Check sheet for the modelled part. Datum: model origin and axes. Units: mm. Round coordinates to 2 decimals unless told otherwise and drop trailing zeros. Loops run counter-clockwise (first coordinate to the right, second up) from the corner with the lowest first, then second, coordinate; pieces in that order, holes last. Notation, with made-up numbers: (-1.75, -35.5) - (7.25, -35.5) arc R19 cw to (7.25, -2.5) - close; hole circle Ø7 at (58.5, 28). An arc over 180 degrees is marked (long way). Answer in a Markdown table with one row per item. Add a question column.
(1) Thickness scan on line 1 along Y through (x, z) = (4, 6.5); line 2 along Y through (x, z) = (-2, 2.5); line 3 along Y through (x, z) = (8.5, 1.25). Record the ranges inside material, lowest first.
(2) Cross-section at C-C on x = -4.5. Enter the section's corners in (y, z).
(3) Cross-section at A-A on x = 12. Enter the section's corners in (y, z).
(4) Cross-section at D-D on x = 0. Enter the section's corners in (y, z).
(5) Gauge pin test, flat ends, axial feed: pin 1 (1.6 mm diameter, centred on x = -13, z = 7, fed in from -Y); pin 2 (3.5 mm diameter, centred on x = 16, z = 6, fed in from +Y); pin 3 (1.9 mm diameter, centred on x = 4, z = 4, fed in from +Y); pin 4 (1 mm diameter, centred on x = 15.5, y = -29, fed in from +Z). Record the tip position at first contact, or that the pin passes through.
Solid Edge part; units mm, degrees
sketch "Sketch1" plane through (0, 0, 0) normal (0, 0, 1) x (1, 0, 0)
  line L0 (-17.9, -27.5) -> (17.9, -27.5)
  line L1 (17.9, -27.5) -> (17.9, 27.5)
  line L2 (17.9, 27.5) -> (-17.9, 27.5)
  line L3 (-17.9, 27.5) -> (-17.9, -27.5)
extrude "Protrusion1" add sketch "Sketch1" along normal blind 8
sketch "Sketch2" plane through (0, -27.5, 4) normal (0, -1, 0) x (1, 0, 0)
  line L0 (-11.1, 0.8) -> (-17.9, 0.8)
  line L1 (-17.9, 0.8) -> (-17.9, -4)
  line L2 (-17.9, -4) -> (-11.1, -4)
  line L3 (-11.1, -4) -> (-11.1, 0.8)
  line L4 (11.1, 0.8) -> (17.9, 0.8)
  line L5 (17.9, 0.8) -> (17.9, -4)
  line L6 (17.9, -4) -> (11.1, -4)
  line L7 (11.1, -4) -> (11.1, 0.8)
extrude "ExtrudedProtrusion_2" add sketch "Sketch2" along normal blind 3.5
sketch "Sketch3" plane through (0, 27.5, 4) normal (0, 1, 0) x (-1, 0, 0)
  line L0 (-17.9, 0.8) -> (-11.1, 0.8)
  line L1 (-11.1, 0.8) -> (-11.1, -4)
  line L2 (-11.1, -4) -> (-17.9, -4)
  line L3 (-17.9, -4) -> (-17.9, 0.8)
  line L4 (11.1, 0.8) -> (17.9, 0.8)
  line L5 (17.9, 0.8) -> (17.9, -4)
  line L6 (17.9, -4) -> (11.1, -4)
  line L7 (11.1, -4) -> (11.1, 0.8)
extrude "ExtrudedProtrusion_3" add sketch "Sketch3" along normal blind 3.5
sketch "Sketch4" plane through (0, 0, 8) normal (0, 0, 1) x (-1, 0, 0)
  line L0 (1.5998, -27.5) -> (1.5998, -24.4524)
  arc A0 (1.5998, -24.4524) -> (2.725, -23) centre (1.225, -23) ccw
  line L1 (2.725, -23) -> (2.725, -21.5)
  arc A1 (2.725, -21.5) -> (1.5998, -20.0476) centre (1.225, -21.5) ccw
  arc A2 (-2.725, -21.5) -> (-1.5998, -20.0476) centre (-1.225, -21.5) cw
  line L2 (-2.725, -23) -> (-2.725, -21.5)
  arc A3 (-1.6, -24.4524) -> (-2.725, -23) centre (-1.225, -23) cw
  line L3 (-1.6, -27.5) -> (-1.6, -24.4524)
  line L4 (0, -27.5) -> (-1.6, -27.5)
  line L5 (0, -27.5) -> (1.5998, -27.5)
  arc A4 (-1.5998, -20.0476) -> (1.5998, -20.0476) centre (0, -20.0254) cw
extrude "ExtrudedCutout_1" cut sketch "Sketch4" against normal blind 8
sketch "Sketch5" plane through (0, 0, 8) normal (0, 0, 1) x (-1, 0, 0)
  line L0 (11.1, 27.5) -> (7.9, 27.5)
  arc A0 (11.1, 27.5) -> (7.9, 27.5) centre (9.5, 27.5) cw
  line L1 (-11.1, 27.5) -> (-7.9, 27.5)
  arc A1 (-7.9, 27.5) -> (-11.1, 27.5) centre (-9.5, 27.5) cw
  arc A2 (-7.9, -27.5) -> (-11.1, -27.5) centre (-9.5, -27.5) ccw
  line L2 (-11.1, -27.5) -> (-7.9, -27.5)
  arc A3 (11.1, -27.5) -> (7.9, -27.5) centre (9.5, -27.5) ccw
  line L3 (11.1, -27.5) -> (7.9, -27.5)
extrude "ExtrudedCutout_2" cut sketch "Sketch5" against normal blind 8
sketch "Sketch6" plane through (0, 0, 8) normal (0, 0, 1) x (-1, 0, 0)
  arc A0 (-1.6, 24.4524) -> (-2.725, 23) centre (-1.225, 23) ccw
  line L0 (-2.725, 23) -> (-2.725, 21.5)
  arc A1 (-2.725, 21.5) -> (-1.5998, 20.0476) centre (-1.225, 21.5) ccw
  arc A2 (-1.5998, 20.0476) -> (1.5998, 20.0476) centre (0, 20.0254) ccw
  arc A3 (2.725, 21.5) -> (1.5998, 20.0476) centre (1.225, 21.5) cw
  line L1 (2.725, 23) -> (2.725, 21.5)
  arc A4 (1.5998, 24.4524) -> (2.725, 23) centre (1.225, 23) cw
  line L2 (1.5998, 27.5) -> (1.5998, 24.4524)
  line L3 (0, 27.5) -> (1.5998, 27.5)
  line L4 (0, 27.5) -> (-1.6, 27.5)
  line L5 (-1.6, 27.5) -> (-1.6, 24.4524)
extrude "Cutout1" cut sketch "Sketch6" against normal up to next
properties material "Polycarbonate"
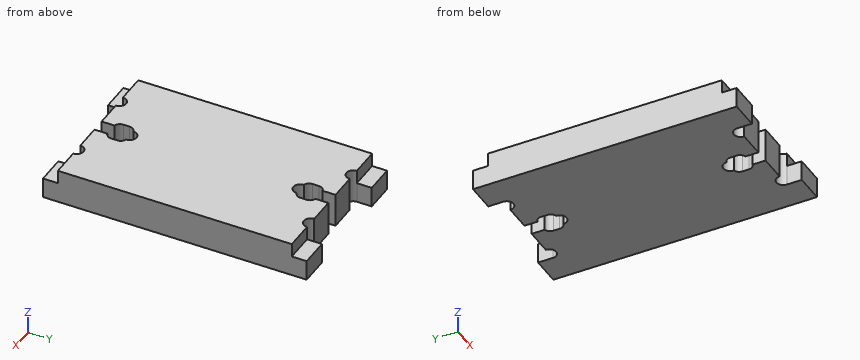
Answers:
| question | item | result |
|---|---|---|
| 1 | line 1 | y = -27.5 to 27.5 |
| 1 | line 2 | y = -27.5 to -24.28, -20.22 to 20.22, 24.28 to 27.5 |
| 1 | line 3 | y = -26.25 to 26.25 |
| 2 | outline | (-27.5, 0) - (27.5, 0) - (27.5, 8) - (-27.5, 8) - close |
| 3 | outline | (-31, 0) - (31, 0) - (31, 4.8) - (27.5, 4.8) - (27.5, 8) - (-27.5, 8) - (-27.5, 4.8) - (-31, 4.8) - close |
| 4 | outline | (-18.43, 0) - (18.43, 0) - (18.43, 8) - (-18.43, 8) - close |
| 5 | pin 1 | stops at y = -27.5 |
| 5 | pin 2 | stops at y = 31 |
| 5 | pin 3 | stops at y = 27.5 |
| 5 | pin 4 | stops at z = 4.8 |
